CAD build for the part. Positions are in the model's coordinates, mm. A direction names the side the tool comes from. Give positions to 0.01 mm unless a question says otherwise; leave off trailing zeros. Order: outer loops, then holes, each group sorted by start corner. A loop starts at its lowest first (then second) coordinate and runs counter-clockwise, first axis right, second up. Notation, with made-up numbers: M -24,84.5 L -6,84.5 A20 cw -6,108.5 Z; hole C 71.5,15.25 d2. An arc over 180 degrees is marked long. Put each result on its own line as item: value. Start each with the question number.
1) Cut at C-C (z = 2.6). Give the number of separate pieces and of enclosed holes in the cut face, and give its area (3 significant figures).
2) Cut at D-D (x = -46.5). Write the cut outline in (y, z).
3) Tool access for faces 1 (the face through (65.917, 14.391, 2.348)), 2 (the face through (-33, 22.462, 2)), 3 (the face through (-34, -22.462, 2)), 4 (the face through (-68.87, 26.17, 2.35)), 5 (the face through (-65.95, 14.47, 2.35)): list every direction of +Z, -Z, +X, -X, +Y, -Y with a clear straight run to the whole face (end or side of a thin tool).
4) Pin check, flat tips, straight feed: pin 1 (2.5 mm diameter, centred on x = 31, z = 2, fed in from +Y); pin 2 (2 mm diameter, centred on y = 25, z = 1.5, fed in from +X); pin 3 (3.5 mm diameter, centred on x = 0, y = -26.37, fed in from -Z); pin 4 (1.4 mm diameter, centred on y = 1, z = 2.5, fed in from -X) (3 decimals). Stop position of each tip, or through.
5) Cut at B-B (y = 8). Write the cut outline in (x, z) (1 decimal), and give its area (3 significant figures).
6) Cut at A-A (x = 0). Write the cut outline in (y, z).
7) Drill centre lines: line 1 (Y direction, x = 0, z = 2.85); line 2 (Y direction, x = -0.5, z = 4.2); line 3 (X direction, y = -21, z = 3.9). Where is each one in solid material? Low to high. Write a range as [from, to].
8) Two-plate mould, pull along X, no slides. Class faces 6 (the face through (-0.1, -31.87, 2.35)), 7 (the face through (-65.325, 0, 2)), 8 (the face through (65.325, 0, 2)), 9 (the face through (0.49, -28.57, 2.35)): released by +X, released by -X, zero draft, split by the parting line, or undercut.
```python
from build123d import *

# Parameters (mm, degrees)
BOSS_EXTRUDE1_DEPTH  = 4.7625
M4_CLEARANCE_HOLE1_D = 4.5


with BuildPart() as part:
    # Sketch1 → Boss-Extrude1 (new body)
    with BuildSketch(Plane.XY):
        with BuildLine():
            Line((61.173729563, 26.089404156), (59.889971157, 24.805645751))
            ThreePointArc((59.889971157, 24.805645751), (57.294584367, 23.07146374), (54.233116908, 22.4625))
            Line((54.233116908, 22.4625), (12.865436095, 22.4625))
            ThreePointArc((12.865436095, 22.4625), (8.142674818, 24.005292715), (5.241473965, 28.038618519))
            ThreePointArc((5.241473965, 28.038618519), (0, 31.8722), (-5.241473965, 28.038618519))
            ThreePointArc((-5.241473965, 28.038618519), (-8.142674818, 24.005292715), (-12.865436095, 22.4625))
            Line((-12.865436095, 22.4625), (-54.233116908, 22.4625))
            ThreePointArc((-54.233116908, 22.4625), (-57.294584367, 23.07146374), (-59.889971157, 24.805645751))
            Line((-59.889971157, 24.805645751), (-61.173729563, 26.089404156))
            ThreePointArc((-61.173729563, 26.089404156), (-68.951904156, 26.089404156), (-68.951904156, 18.311229563))
            Line((-68.951904156, 18.311229563), (-67.668145751, 17.027471157))
            ThreePointArc((-67.668145751, 17.027471157), (-65.93396374, 14.432084367), (-65.325, 11.370616908))
            Line((-65.325, 11.370616908), (-65.325, -11.370616908))
            ThreePointArc((-65.325, -11.370616908), (-65.93396374, -14.432084367), (-67.668145751, -17.027471157))
            Line((-67.668145751, -17.027471157), (-68.951904156, -18.311229563))
            ThreePointArc((-68.951904156, -18.311229563), (-68.951904156, -26.089404156), (-61.173729563, -26.089404156))
            Line((-61.173729563, -26.089404156), (-59.889971157, -24.805645751))
            ThreePointArc((-59.889971157, -24.805645751), (-57.294584367, -23.07146374), (-54.233116908, -22.4625))
            Line((-54.233116908, -22.4625), (-12.865436095, -22.4625))
            ThreePointArc((-12.865436095, -22.4625), (-8.142674818, -24.005292715), (-5.241473965, -28.038618519))
            ThreePointArc((-5.241473965, -28.038618519), (0, -31.8722), (5.241473965, -28.038618519))
            ThreePointArc((5.241473965, -28.038618519), (8.142674818, -24.005292715), (12.865436095, -22.4625))
            Line((12.865436095, -22.4625), (54.233116908, -22.4625))
            ThreePointArc((54.233116908, -22.4625), (57.294584367, -23.07146374), (59.889971157, -24.805645751))
            Line((59.889971157, -24.805645751), (61.173729563, -26.089404156))
            ThreePointArc((61.173729563, -26.089404156), (68.951904156, -26.089404156), (68.951904156, -18.311229563))
            Line((68.951904156, -18.311229563), (67.668145751, -17.027471157))
            ThreePointArc((67.668145751, -17.027471157), (65.93396374, -14.432084367), (65.325, -11.370616908))
            Line((65.325, -11.370616908), (65.325, 11.370616908))
            ThreePointArc((65.325, 11.370616908), (65.93396374, 14.432084367), (67.668145751, 17.027471157))
            Line((67.668145751, 17.027471157), (68.951904156, 18.311229563))
            ThreePointArc((68.951904156, 18.311229563), (68.951904156, 26.089404156), (61.173729563, 26.089404156))
        make_face()
    extrude(amount=BOSS_EXTRUDE1_DEPTH)

    # M4 Clearance Hole1 (through all)
    with Locations(Plane.XY.offset(4.7625)):
        with Locations((-65.062816859, 22.200316859), (0, 26.3722), (65.062816859, 22.200316859), (65.062816859, -22.200316859), (0, -26.3722), (-65.062816859, -22.200316859)):
            Hole(M4_CLEARANCE_HOLE1_D / 2)


solid = part.part
```
Solution:
1. separate pieces: 1
1. enclosed holes: 6
1. area: 6,300 mm²
2. outline: M -22.46,0 L 22.46,0 L 22.46,4.76 L -22.46,4.76 Z
3. face 1: +Z, -Z, +X
3. face 2: +Z, -Z, +Y
3. face 3: +Z, -Z, -Y
3. face 4: +Z, -Z
3. face 5: +Z, -Z, -X
4. pin 1: y = 22.46
4. pin 2: x = 70.26
4. pin 3: through
4. pin 4: x = -65.325
5. outline: M -65.3,0 L 65.3,0 L 65.3,4.8 L -65.3,4.8 Z
5. area: 622 mm²
6. outline: M -31.87,0 L -28.62,0 L -28.62,4.76 L -31.87,4.76 Z; M -24.12,0 L 24.12,0 L 24.12,4.76 L -24.12,4.76 Z; M 28.62,0 L 31.87,0 L 31.87,4.76 L 28.62,4.76 Z
7. line 1: [-31.87, -28.62], [-24.12, 24.12], [28.62, 31.87]
7. line 2: [-31.85, -28.57], [-24.18, 24.18], [28.57, 31.85]
7. line 3: [-70.43, -66.97], [-63.16, 63.16], [66.97, 70.43]
8. face 6: split by the parting line
8. face 7: released by -X
8. face 8: released by +X
8. face 9: undercut
